Input: part model. Units: mm. Frame: model coordinates. Face numbers are marked on the shaded views. A direction names the side the tool comes from. Round coordinates to 2 decimals unless told otherwise and drop trailing zeros. Loops run counter-clockwise (first coordinate to the right, second up) from the corner with the lowest first, then second, coordinate; pieces in that order, holes last.
(1) First-contact query: pin 1 Ø18 at (y, z) = (21, 13) entering from +X; pin 2 Ø8 at (x, y) = (25, 11) entering from -Z; pin 3 Ø12 at (x, z) = (44.5, 22) entering from +Y; pin 4 Ø8 at (y, z) = (42.902, 9.483) entering from +X. Flat tips, straight axial feed; report the tip coordinate or a pass-through.
(2) Access query for the marked faces 1, 2 and 3. Directions: +Z, -Z, +X, -X, +Y, -Y. A direction counts if a zero-diameter tool reaches every point of the face in a straight line with its end or side. Return the directions, or none.
(3) Draft query along Y for the marked faces 4, 5 and 6. Return one class per face: released by +Y, released by -Y, zero draft, split by the parting line, or undercut.
(4) Cut plane A-A, the plane z = 13. Output: boundary loops of the cut face in (x, y).
(5) Cut plane D-D, the plane y = 47. Output: boundary loops of the cut face in (x, z).
(6) Line query: line 1 (X direction, y = 15.5, z = 4); line 2 (Y direction, x = 37, z = 16.5); line 3 (X direction, y = 17.5, z = 29). Output: solid intervals per line, ascending.
(7) Cut plane B-B, the plane y = 25. Output: boundary loops of the cut face in (x, z).
(8) Cut plane C-C, the plane x = 26. Output: boundary loops of the cut face in (y, z).
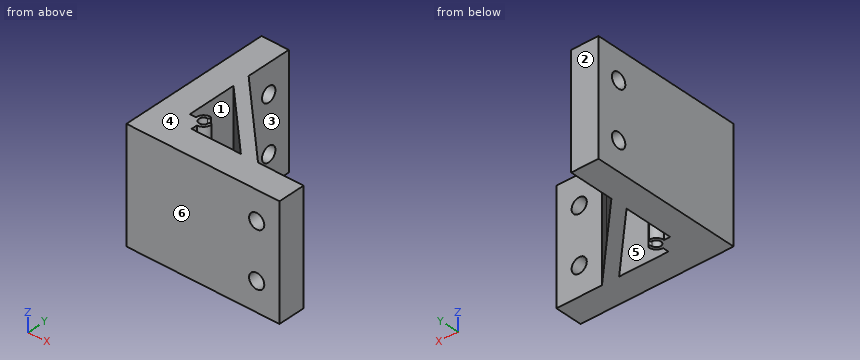
from build123d import *

# Parameters (mm, degrees)
BOSS_EXTRUDE2_DEPTH = 37
BOSS_EXTRUDE3_DEPTH = 37
CUT_EXTRUDE1_REACH  = 76.99
SKETCH2_R           = 2.5


with BuildPart() as part:
    # Sketch1 → Boss-Extrude2 (new body)
    with BuildSketch(Plane.XY):
        with BuildLine():
            Line((0, 50.402000333), (0, 0))
            Line((0, 0), (11.732233047, 11.732233047))
            ThreePointArc((11.732233047, 11.732233047), (11.190301169, 12.543291419), (11, 13.5))
            Line((11, 13.5), (9, 13.5))
            Line((9, 13.5), (9, 29.745146084))
            Line((9, 29.745146084), (19.372573042, 19.372573042))
            Line((19.372573042, 19.372573042), (22.201000167, 22.201000167))
            Line((22.201000167, 22.201000167), (9, 35.402000333))
            Line((9, 35.402000333), (9, 50.402000333))
            Line((9, 50.402000333), (0, 50.402000333))
        make_face()
        with BuildLine():
            Line((11.732233047, 11.732233047), (0, 0))
            Line((0, 0), (50.402000333, 0))
            Line((50.402000333, 0), (50.402000333, 9))
            Line((50.402000333, 9), (35.402000333, 9))
            Line((35.402000333, 9), (22.201000167, 22.201000167))
            Line((22.201000167, 22.201000167), (19.372573042, 19.372573042))
            Line((19.372573042, 19.372573042), (29.745146084, 9))
            Line((29.745146084, 9), (13.5, 9))
            Line((13.5, 9), (13.5, 11))
            ThreePointArc((13.5, 11), (12.543291419, 11.190301169), (11.732233047, 11.732233047))
        make_face()
    extrude(amount=BOSS_EXTRUDE2_DEPTH)

    # Sketch1_4 → Boss-Extrude3 (add)
    with BuildSketch(Plane.XY):
        with BuildLine():
            ThreePointArc((13.5, 16), (11.732233047, 11.732233047), (16, 13.5))
            ThreePointArc((16, 13.5), (15.5, 14), (15, 13.5))
            ThreePointArc((15, 13.5), (12.439339828, 12.439339828), (13.5, 15))
            ThreePointArc((13.5, 15), (14, 15.5), (13.5, 16))
        make_face()
    extrude(amount=BOSS_EXTRUDE3_DEPTH)

    # Sketch2 → Cut-Extrude1 (cut, up to next)
    with BuildSketch(Plane(origin=(9, 0, 0), x_dir=(0, 0, -1), z_dir=(1, 0, 0)), mode=Mode.PRIVATE) as cut_extrude1_sk1:
        with Locations(Location((-27.517, 42.902000333, 0), (0, 0, 90))):
            Circle(SKETCH2_R)
    cut_extrude1_tool1 = extrude(cut_extrude1_sk1.sketch, amount=-CUT_EXTRUDE1_REACH, mode=Mode.PRIVATE) & part.part
    # Sketch2 → Cut-Extrude1 (cut, up to next)
    with BuildSketch(Plane(origin=(9, 0, 0), x_dir=(0, 0, -1), z_dir=(1, 0, 0)), mode=Mode.PRIVATE) as cut_extrude1_sk2:
        with Locations(Location((-9.483, 42.902000333, 0), (0, 0, 90))):
            Circle(SKETCH2_R)
    cut_extrude1_tool2 = extrude(cut_extrude1_sk2.sketch, amount=-CUT_EXTRUDE1_REACH, mode=Mode.PRIVATE) & part.part
    cut_extrude1_1 = cut_extrude1_tool1.solids().sort_by_distance((9, 42.902, 27.517))[0]
    add(cut_extrude1_1, mode=Mode.SUBTRACT)
    cut_extrude1_2 = cut_extrude1_tool2.solids().sort_by_distance((9, 42.902, 9.483))[0]
    add(cut_extrude1_2, mode=Mode.SUBTRACT)
    cut_extrude1 = cut_extrude1_1 + cut_extrude1_2  # Cut-Extrude1 as one shape, for the pattern or mirror that repeats it

    # Mirror1: Cut-Extrude1 across plane
    add(cut_extrude1.mirror(Plane(origin=(0, 0, 0), x_dir=(0, 0, 1), z_dir=(0.7071067811865464, -0.7071067811865488, 0))), mode=Mode.SUBTRACT)


solid = part.part
Reported:
1. pin 1: stops at x = 32.4
1. pin 2: stops at z = 0
1. pin 3: stops at y = 9
1. pin 4: stops at x = 9
2. face 1: +Z, -Z
2. face 2: +Z, -Z, +X, -X, +Y
2. face 3: +Z, -Z, +X, +Y
3. face 4: zero draft
3. face 5: undercut
3. face 6: released by -Y
4. outline: (0, 0) - (50.4, 0) - (50.4, 9) - (35.4, 9) - (9, 35.4) - (9, 50.4) - (0, 50.4) - close; hole (9, 13.5) - (11, 13.5) arc R2.5 cw to (13.5, 16) arc R0.5 cw to (13.5, 15) arc R1.5 ccw (long way) to (15, 13.5) arc R0.5 cw to (16, 13.5) arc R2.5 cw to (13.5, 11) - (13.5, 9) - (29.75, 9) - (9, 29.75) - close
5. outline: (0, 0) - (9, 0) - (9, 37) - (0, 37) - close
6. line 1: x = 0 to 9, 12 to 14, 23.25 to 28.9
6. line 2: y = 0 to 9
6. line 3: x = 0 to 9, 21.25 to 26.9
7. outline: (0, 0) - (9, 0) - (9, 37) - (0, 37) - close; (13.75, 0) - (19.4, 0) - (19.4, 37) - (13.75, 37) - close
8. outline: (0, 0) - (9, 0) - (9, 37) - (0, 37) - close; (12.75, 0) - (18.4, 0) - (18.4, 37) - (12.75, 37) - close
